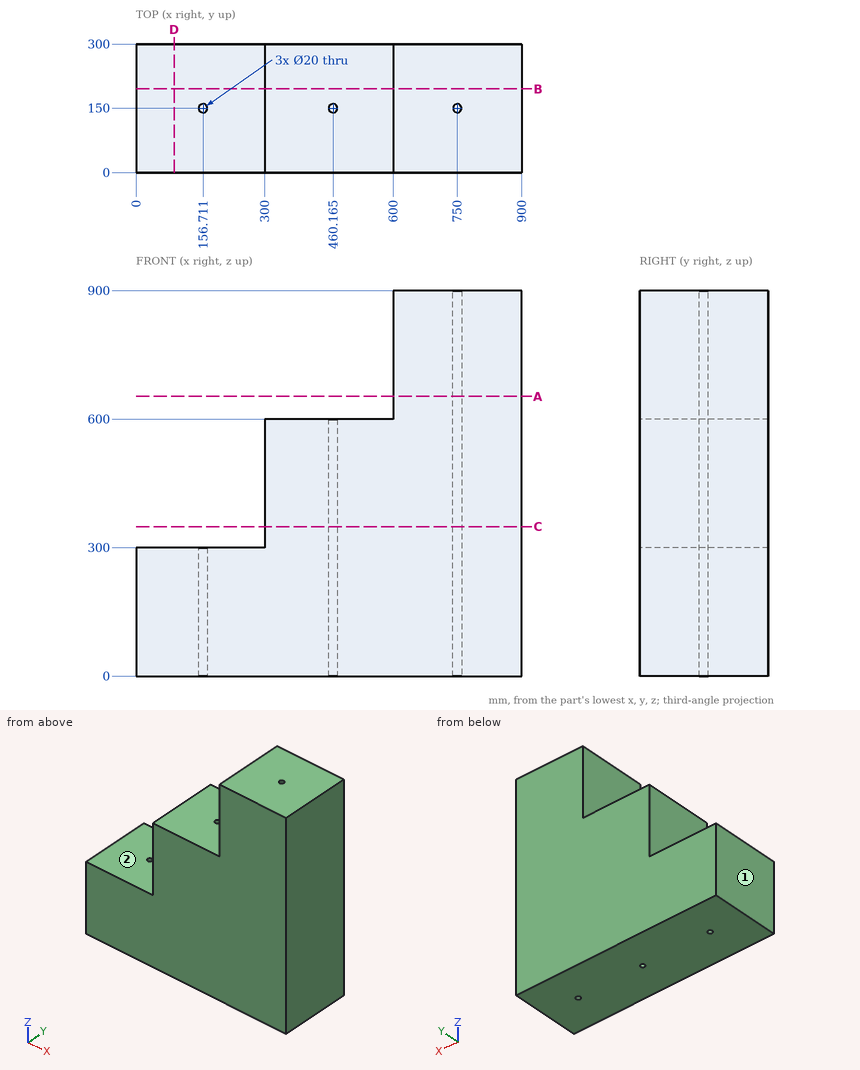
For this review, use the dimensioned drawing (mm, ordinates from the lowest corner) and the shaded views. A direction names the side the tool comes from. Coordinates: 2 decimals unless noted, no trailing zeros. Order: outer loops, then holes, each group sorted by start corner. A loop starts at its lowest first (then second) coordinate and runs counter-clockwise, first axis right, second up. Notation, with made-up numbers: (1, 15) - (29, 15) arc R23 cw to (29, 35) - close; hole circle Ø10 at (-38, 38.5). An arc over 180 degrees is marked (long way). Answer in a Markdown table with one row per item.
(1) For the marked faces 1 and 2, list the 3-axis set-ups (+Z, -Z, +X, -X, +Y, -Y) from which the entire face can be reached by the end or side of a thin tool; tool diameter is ignored.
Checked values:
| item | result |
|---|---|
| face 1 | +Z, -Z, -X, +Y, -Y |
| face 2 | +Z, -X, +Y, -Y |
(2) Wall thickness on line 1 along Z through (x, y) = (508.5, 147.5); line 2 along Y through (x, z) = (750, 414); line 3 along X through (y, z) = (217.5, 769.5): over which ranges is each line inside the solid? List them lowest first. Write a range as from..to.
Checked values:
| item | result |
|---|---|
| line 1 | 0..600 |
| line 2 | 0..140, 160..300 |
| line 3 | 600..900 |
(3) Clearance check with flat-ended pins moving along their axes: pin 1 (8 mm diameter, centred on x = 219, y = 147.5, fed in from +Z); pin 2 (18 mm diameter, centred on x = 156.71, y = 150, fed in from -Z); pin 3 (6 mm diameter, centred on y = 236, z = 396.5, fed in from -X). State where each tip first meets the part, or that it passes through.
Checked values:
| item | result |
|---|---|
| pin 1 | z = 300 |
| pin 2 | through |
| pin 3 | x = 300 |
(4) Consider section D-D on x = 89. State the section outline as (y, z) points.
Checked values:
| item | result |
|---|---|
| outline | (0, 0) - (300, 0) - (300, 300) - (0, 300) - close |
(5) Consider section C-C on z = 348.5. State the section outline as (x, y) points (1 decimal), plus the area to 3 significant figures.
Checked values:
| item | result |
|---|---|
| outline | (300, 0) - (900, 0) - (900, 300) - (300, 300) - close; hole circle Ø20 at (460.2, 150); hole circle Ø20 at (750, 150) |
| area | 179,000 mm^2 |
(6) Consider section B-B on y = 195.5. State the section outline as (x, z) points, plus the area to 3 significant figures.
Checked values:
| item | result |
|---|---|
| outline | (0, 0) - (900, 0) - (900, 900) - (600, 900) - (600, 600) - (300, 600) - (300, 300) - (0, 300) - close |
| area | 540,000 mm^2 |
(7) Consider section A-A on z = 653. State the section outline as (x, y) points, plus the area to 3 significant figures.
Checked values:
| item | result |
|---|---|
| outline | (600, 0) - (900, 0) - (900, 300) - (600, 300) - close; hole circle Ø20 at (750, 150) |
| area | 89,700 mm^2 |
